Could you check a few things on this model? Use its own coordinates, in mm. Give positions to 0.01 mm unless a question says otherwise; leave off trailing zeros. Order: outer loops, then holes, each group sorted by start corner. A loop starts at its lowest first (then second) coordinate and runs counter-clockwise, first axis right, second up. Notation, with made-up numbers: M 89,-22.5 L 113,-22.5 A24 cw 113,-0.5 Z; hole C 14.25,77.25 d7. An arc over 180 degrees is marked long. Use a Markdown table: item, result. Add a question column.
```python
from build123d import *

# Parameters (mm, degrees)
F1_DEPTH = 127


with BuildPart() as f1:
    # F0 (on Top) → F1 (new body, symmetric)
    with BuildSketch(Plane.XY):
        with BuildLine():
            ThreePointArc((-33.009991, -22.410832), (-31.150119, -26.90096), (-26.659991, -28.760832))
            Line((-26.659991, -28.760832), (-11.74327, -28.760832))
            ThreePointArc((-11.74327, -28.760832), (6.484724, -10.532838), (24.712717, -28.760832))
            Line((24.712717, -28.760832), (40.160779, -28.760832))
            Line((40.160779, -28.760832), (40.160779, 23.01116))
            ThreePointArc((40.160779, 23.01116), (38.300907, 27.501289), (33.810779, 29.36116))
            Line((33.810779, 29.36116), (-33.009991, 29.36116))
            Line((-33.009991, 29.36116), (-33.009991, -22.410832))
        make_face()
    extrude(amount=F1_DEPTH, both=True)


solid = f1.part
```
1) We'd pull the mould along X, two halves only. Please class faces 1 (the face through (3, 1, -127)), 2 (the face through (6.084, -10.537, 1.778)), 3 (the face through (38.35, 27.45, 1.78)): pulls with the +X half, pulls with the -X half, needs draft (parallel to the pull), parting line crosses it, or undercut.
2) Suppose I cut it at C-C on x = 7.5. Please give me the cut outline in (y, z), and give its area (3 significant figures).
3) Suppose I cut it at B-B on y = -25. Please give me the cut outline in (x, z).
4) Please list where these lines run through material, in increasing order: line 1 (X direction, y = -13, z = -18.5); line 2 (X direction, y = 23.5, z = -99); line 3 (X direction, y = -21, z = 60.5). Write a range as from..to.
Values found:
| question | item | result |
|---|---|---|
| 1 | face 1 | needs draft |
| 1 | face 2 | undercut |
| 1 | face 3 | pulls with the +X half |
| 2 | outline | M -10.56,-127 L 29.36,-127 L 29.36,127 L -10.56,127 Z |
| 2 | area | 10,100 mm^2 |
| 3 | outline | M -32.46,-127 L -11.35,-127 L -11.35,127 L -32.46,127 Z; M 24.32,-127 L 40.16,-127 L 40.16,127 L 24.32,127 Z |
| 4 | line 1 | x = -33.01..-2.67, 15.64..40.16 |
| 4 | line 2 | x = -33.01..40.14 |
| 4 | line 3 | x = -33.01..-10.01, 22.98..40.16 |
